Can you work these out from the drawing? Everything is in mm from the part's minimum corner. A direction names the side the tool comes from. Round coordinates to 2 decimals unless told otherwise and drop trailing zeros. Write each loop counter-clockwise with the first axis right and the second up, starting at its lowest first coordinate (ties: lowest second). Pieces come first, ordered by that corner, then holes. Notation, with made-up numbers: (-18, -10.75) - (33, -10.75) arc R19 ccw to (33, 10.25) - close; hole circle Ø10 at (14.5, 5.25). An arc over 180 degrees is marked (long way). One line per item, written item: value. Start each with the question number.
Item 1: Thinking about a two-plate mould opening in Z: for the marked faces 1, 2 and 3, which applies, released by +Z, released by -Z, zero draft, split by the parting line, or undercut?
Item 2: Imagine slicing it at C-C, the plane z = 7. Please give me the cut outline in (x, y).
Item 3: If I drill on line 1 (Z direction, x = 4.25, y = 1.75); line 2 (X direction, y = 2.5, z = 6.5); line 3 (Y direction, x = 6, z = 1.25), over which ranges is the centre line in solid material (lowest first)?
Item 4: Imagine slicing it at B-B, the plane x = 6. Please give me the cut outline in (y, z), then the cut area to 3 significant figures.
Item 5: Imagine slicing it at A-A, the plane y = 3.5. Please give me the cut outline in (x, z), then the cut area to 3 significant figures.
Item 6: Imagine slicing it at D-D, the plane x = 7.5. Please give me the cut outline in (y, z).
Item 7: For the marked faces 4, 5, 6, 7 and 8, which set-ups out of +Z, -Z, +X, -X, +Y, -Y let a thin tool reach every point of the face, with its end or its side?
Item 8: For P1, Ø2, axis at y = 17, z = 7, coming from the +X side; P2, Ø2, axis at x = 7, y = 3, coming from the -Z side; P3, Ø1.6, axis at y = 1, z = 2.5, coming from the -X side, each with a flat end and sliding along its axis, tell me the tip position at first contact or that it passes through.
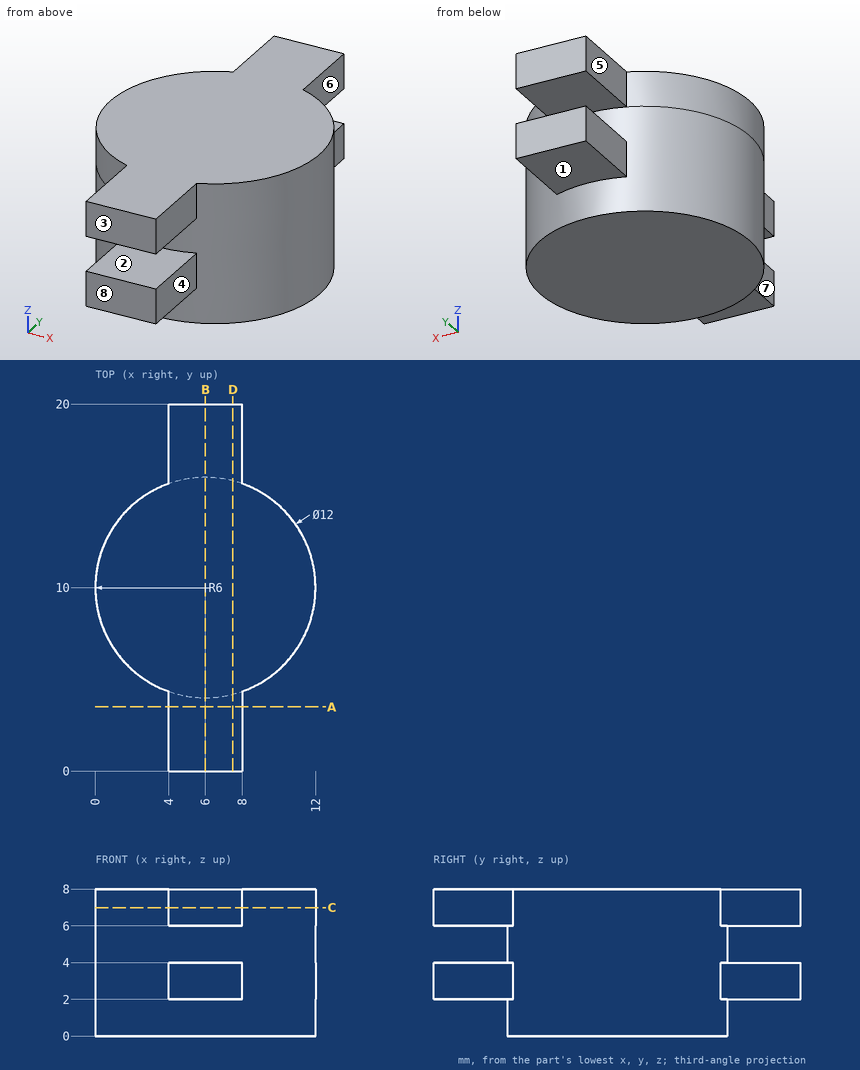
Values follow:
1. face 1: released by -Z
1. face 2: undercut
1. face 3: zero draft
2. outline: (4, 0) - (8, 0) - (8, 4.34) arc R6 ccw to (8, 15.66) - (8, 20) - (4, 20) - (4, 15.66) arc R6 ccw to (4, 4.34) - close
3. line 1: z = 2 to 4, 6 to 8
3. line 2: x = 4 to 8
3. line 3: y = 4 to 16
4. outline: (0, 2) - (4, 2) - (4, 0) - (16, 0) - (16, 2) - (20, 2) - (20, 4) - (16, 4) - (16, 6) - (20, 6) - (20, 8) - (0, 8) - (0, 6) - (4, 6) - (4, 4) - (0, 4) - close
4. area: 128 mm^2
5. outline: (4, 2) - (8, 2) - (8, 4) - (4, 4) - close; (4, 6) - (8, 6) - (8, 8) - (4, 8) - close
5. area: 16.0 mm^2
6. outline: (0, 2) - (4.19, 2) - (4.19, 0) - (15.81, 0) - (15.81, 2) - (20, 2) - (20, 4) - (15.81, 4) - (15.81, 6) - (20, 6) - (20, 8) - (0, 8) - (0, 6) - (4.19, 6) - (4.19, 4) - (0, 4) - close
7. face 4: +Z, -Z, +X, -Y
7. face 5: +Z, -Z, -X, +Y
7. face 6: +Z, -Z, +X, +Y
7. face 7: +Z, -Z, -X, -Y
7. face 8: +Z, -Z, +X, -X, -Y
8. P1: stops at x = 8
8. P2: stops at z = 2
8. P3: stops at x = 4
